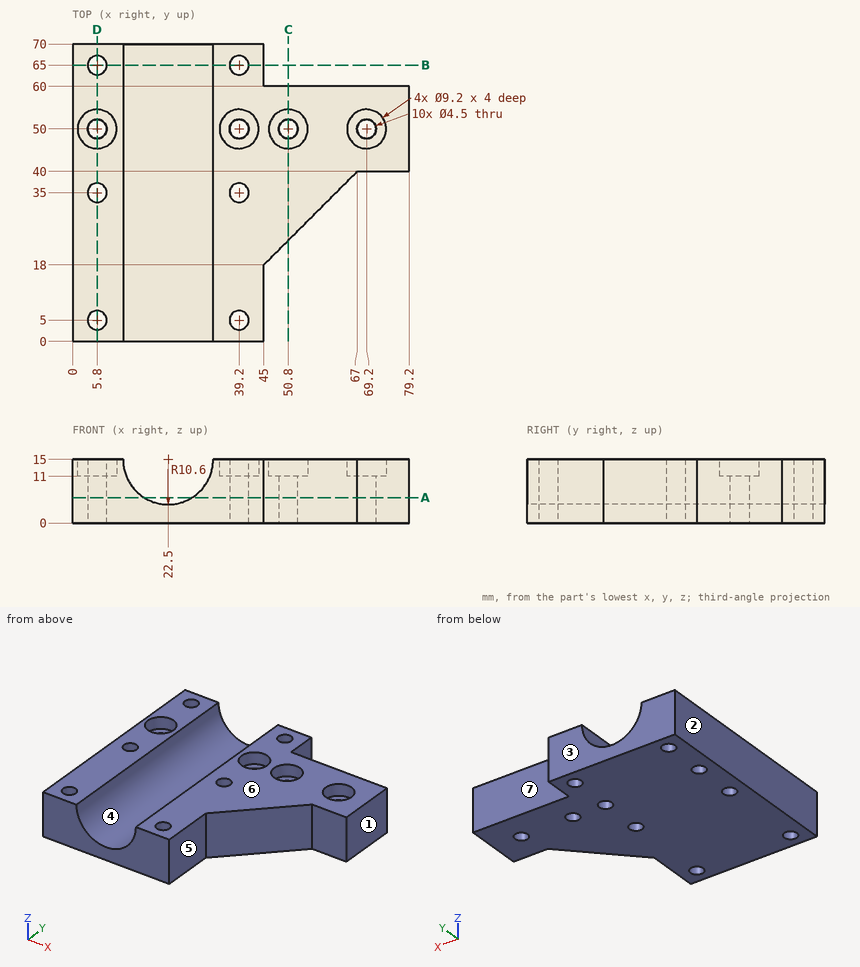
Study the drawing (mm; zero at the part's minimum x, y, z) and answer. A direction names the side the tool comes from. Round coordinates to 2 decimals unless told otherwise and drop trailing zeros. Write each loop counter-clockwise with the first axis right and the second up, starting at its lowest first coordinate (ties: lowest second). Pieces come first, ordered by that corner, then holes. Notation, with made-up numbers: (21.5, -17) -> (37.5, -17) arc R31 cw to (37.5, 14) -> close; hole circle Ø1 at (81, 21). An arc over 180 degrees is marked (long way). Write item = value, one per line.
1) Section C-C on x = 50.8 is taken. Write down the section's boundary in (y, z).
Check values:
outline = (23.8, 0) -> (47.75, 0) -> (47.75, 11) -> (45.4, 11) -> (45.4, 15) -> (23.8, 15) -> close; (52.25, 0) -> (60, 0) -> (60, 15) -> (54.6, 15) -> (54.6, 11) -> (52.25, 11) -> close
2) Section A-A on z = 6 is taken. Give the number of separate pieces and of enclosed holes in the cut face, plus the area to 3 significant figures.
Check values:
separate_pieces = 2
enclosed_holes = 10
area = 3,130 mm²
3) For a pull along X with two mould halves and no side action, classify the marked faces 1, 2, 3 and 4 as released by +X, released by -X, zero draft, split by the parting line, or undercut.
Check values:
face_1 = released by +X
face_2 = released by -X
face_3 = zero draft
face_4 = undercut
4) Straight lines are drawn through the part: line 1 along Y through (x, z) = (39.2, 6); line 2 along X through (y, z) = (50, 4.25); line 3 along X through (y, z) = (37, 10.5). For each, find the intervals that lie inside material, in ascending order. Write a range as [from, to].
Check values:
line_1 = [0, 2.75], [7.25, 32.75], [37.25, 47.75], [52.25, 62.75], [67.25, 70]
line_2 = [0, 3.55], [8.05, 36.95], [41.45, 48.55], [53.05, 66.95], [71.45, 79.2]
line_3 = [0, 4.77], [6.83, 12.9], [32.1, 38.17], [40.23, 64]
5) Section B-B on y = 65 is taken. Write down the section's boundary in (x, z).
Check values:
outline = (0, 0) -> (3.55, 0) -> (3.55, 15) -> (0, 15) -> close; (8.05, 0) -> (36.95, 0) -> (36.95, 15) -> (33.1, 15) arc R10.6 cw to (11.9, 15) -> (8.05, 15) -> close; (41.45, 0) -> (45, 0) -> (45, 15) -> (41.45, 15) -> close
6) Which of the six approach directions +Z, -Z, +X, -X, +Y, -Y give full straight-line access (tool end or side, diameter ignored) to the marked faces 5, 6 and 7?
Check values:
face_5 = +Z, -Z, +X, -Y
face_6 = +Z, +X, -X, +Y, -Y
face_7 = +Z, -Z, +X, +Y
7) Section D-D on x = 5.8 is taken. Write down the section's boundary in (y, z), plus the area to 3 significant figures.
Check values:
outline = (0, 0) -> (2.75, 0) -> (2.75, 15) -> (0, 15) -> close; (7.25, 0) -> (32.75, 0) -> (32.75, 15) -> (7.25, 15) -> close; (37.25, 0) -> (47.75, 0) -> (47.75, 11) -> (45.4, 11) -> (45.4, 15) -> (37.25, 15) -> close; (52.25, 0) -> (62.75, 0) -> (62.75, 15) -> (54.6, 15) -> (54.6, 11) -> (52.25, 11) -> close; (67.25, 0) -> (70, 0) -> (70, 15) -> (67.25, 15) -> close
area = 761 mm²
8) Given pin 1 (3 mm diameter, centred on x = 27, y = 21.5, fed in from -Z); pin 2 (3 mm diameter, centred on y = 23, z = 3.5, fed in from +X); pin 3 (4 mm diameter, centred on x = 5.8, y = 65, fed in from -Z); pin 4 (6 mm diameter, centred on x = 76, z = 8, fed in from -Y), each flat-ended and moving along its own axis, determine where each tip first touches the part or whether it passes through.
Check values:
pin_1 = 0
pin_2 = 51.5
pin_3 = through
pin_4 = 40
